Read the model definition and answer for the solid it produces. Units are mm, in the model's axes. A direction names the side the tool comes from. Coordinates: 2 decimals unless noted, no trailing zeros. Order: outer loops, then holes, each group sorted by start corner. A loop starts at its lowest first (then second) coordinate and runs counter-clockwise, first axis right, second up. Notation, with made-up numbers: (25.5, 63.5) -> (75.5, 63.5) arc R29 cw to (75.5, 86.5) -> close; hole circle Ø5 at (68.5, 51.25). An arc over 180 degrees is marked (long way). Return JSON: item names as keys, results as strings. Group by question number.
```python
from build123d import *

# Parameters (mm, degrees)
ESQUISSE1_R             = 65
DISQUE_DEPTH            = 3
ESQUISSE3_W             = 30.466369815
ESQUISSE3_H             = 200
COT_S_DEPTH             = 4
D_GAGEMENT_M42_D        = 4.5
ESQUISSE15_W            = 89.863216067
ESQUISSE15_H            = 32.096215679
ENL_V_MAT_EXTRU_1_DEPTH = 4
EMPLACEMENT_COMPOS_W    = 48
EMPLACEMENT_COMPOS_H    = 19
EMPLACEMENT_COMPOS_W_2  = 65
EMPLACEMENT_COMPOS_W_3  = 120.200529509
EMPLACEMENT_COMPOS_H_2  = 30.626013932
ENL_V_MAT_EXTRU_2_DEPTH = 4
CONG_1_R                = 8
D_GAGEMENT_M3_51_D      = 3.9
D_GAGEMENT_M3_51_DEPTH  = 3
D_GAGEMENT_M3_51_TIP    = 1.171678207
ESQUISSE19_W            = 20.5
ESQUISSE19_H            = 24.73475383
ENL_V_MAT_EXTRU_3_DEPTH = 4
ESQUISSE22_W            = 15
ESQUISSE22_H            = 22.73475383
ENL_V_MAT_EXTRU_4_DEPTH = 4


with BuildPart() as part:
    # Esquisse1 → disque (new body)
    with BuildSketch(Plane(origin=(0, 0, 0), x_dir=(1, 0, 0), z_dir=(0, 1, 0))):
        Circle(ESQUISSE1_R)
    extrude(amount=DISQUE_DEPTH)

    # Esquisse3 → cotés (cut, through all)
    with BuildSketch(Plane(origin=(0, 3, 0), x_dir=(1, 0, 0), z_dir=(0, 1, 0))):
        with Locations((-55.233184908, 0)):
            Rectangle(ESQUISSE3_W, ESQUISSE3_H)
        with Locations((55.233184908, 0)):
            Rectangle(ESQUISSE3_W, ESQUISSE3_H)
    extrude(amount=-COT_S_DEPTH, mode=Mode.SUBTRACT)

    # Dégagement M42 (through all)
    with Locations(Plane(origin=(0, 3, 0), x_dir=(1, 0, 0), z_dir=(0, 1, 0))):
        with Locations((-32.5, 42.5), (32.5, 42.5), (32.5, -42.5), (-32.5, -42.5)):
            Hole(D_GAGEMENT_M42_D / 2)

    # Esquisse15 → Enlèv. mat.-Extru.1 (cut, through all)
    with BuildSketch(Plane.XZ):
        with Locations((-4.931608034, 67.282861669)):
            Rectangle(ESQUISSE15_W, ESQUISSE15_H)
    extrude(amount=-ENL_V_MAT_EXTRU_1_DEPTH, mode=Mode.SUBTRACT)

    # emplacement compos → Enlèv. mat.-Extru.2 (cut, through all)
    with BuildSketch(Plane(origin=(0, 0, 0), x_dir=(-1, 0, 0), z_dir=(0, -1, 0))):
        with Locations((0, 38.367376915)):
            Rectangle(EMPLACEMENT_COMPOS_W, EMPLACEMENT_COMPOS_H)
        with Locations((0, 16)):
            Rectangle(EMPLACEMENT_COMPOS_W_2, EMPLACEMENT_COMPOS_H)
        with Locations((-20.100264755, 66.547760796)):
            Rectangle(EMPLACEMENT_COMPOS_W_3, EMPLACEMENT_COMPOS_H_2)
    extrude(amount=-ENL_V_MAT_EXTRU_2_DEPTH, mode=Mode.SUBTRACT)

    # Congé1
    cong_1_edges = [part.edges().sort_by_distance(p)[0] for p in [
        (40, 1.5, -51.23475383),
        (40, 1.5, 51.23475383),
        (-40, 1.5, 51.23475383),
        (-40, 1.5, -51.23475383),
    ]]
    fillet(cong_1_edges, radius=CONG_1_R)

    # Dégagement M3.51
    with Locations(Plane(origin=(0, 3, 0), x_dir=(1, 0, 0), z_dir=(0, 1, 0))):
        with Locations((-7.5, -28.23475383), (7.5, -28.23475383), (7.5, -43.23475383), (-7.5, -43.23475383)):
            Hole(D_GAGEMENT_M3_51_D / 2, depth=D_GAGEMENT_M3_51_DEPTH)
            with Locations((0, 0, -(D_GAGEMENT_M3_51_DEPTH + D_GAGEMENT_M3_51_TIP / 2))):  # 118° drill point
                Cone(0, D_GAGEMENT_M3_51_D / 2, D_GAGEMENT_M3_51_TIP, mode=Mode.SUBTRACT)

    # Esquisse19 → Enlèv. mat.-Extru.3 (cut, through all)
    with BuildSketch(Plane(origin=(0, 3, 0), x_dir=(1, 0, 0), z_dir=(0, 1, 0))):
        with Locations((-22.75, -10.867376915)):
            Rectangle(ESQUISSE19_W, ESQUISSE19_H)
    enl_v_mat_extru_3 = extrude(amount=-ENL_V_MAT_EXTRU_3_DEPTH, mode=Mode.SUBTRACT)

    # Symétrie1: Enlèv. mat.-Extru.3 across plane
    add(enl_v_mat_extru_3.mirror(Plane.ZY), mode=Mode.SUBTRACT)

    # Esquisse22 → Enlèv. mat.-Extru.4 (cut, through all)
    with BuildSketch(Plane(origin=(0, 3, 0), x_dir=(1, 0, 0), z_dir=(0, 1, 0))):
        with Locations((0, -9.867376915)):
            Rectangle(ESQUISSE22_W, ESQUISSE22_H)
    extrude(amount=-ENL_V_MAT_EXTRU_4_DEPTH, mode=Mode.SUBTRACT)


solid = part.part
```
1. Find section D-D on z = -10. Determine the outline of the cut face in (x, y).
2. Find section B-B on z = 6. Determine the outline of the cut face in (x, y).
3. Find section C-C on x = 20.5. Determine the outline of the cut face in (y, z), and give its area (3 significant figures).
4. Find section A-A on z = -32.5. Determine the outline of the cut face in (x, y).
5. Given pin 1 (2.5 mm diameter, centred on x = 32.5, z = 42.5, fed in from +Y), flat-ended and moving along its own axis, determine where the tip first touches the part or whether it passes through.
6. Which of the six approach directions +Z, -Z, +X, -X, +Y, -Y give full straight-line access (tool end or side, diameter ignored) to faces 1 (the face through (23, 2, -1.5)), 2 (the face through (37.594, 1.479, -48.953))?
7. For a pull along Z with two mould halves and no side action, classify faces 3 (the face through (-37.72, 1.48, 48.83)), 4 (the face through (-33.71, 1.479, 40.603)), 5 (the face through (-9, 3, 11)), 6 (the face through (7.5, 2, 10)) as released by +Z, released by -Z, zero draft, split by the parting line, or undercut.
8. Straight lines are drawn through the part: L1, parallel to X at y = 1.3, z = 9.5; L2, parallel to Z at x = -12, y = 0.85; L3, parallel to Z at x = -17, y = 2.75. For each, find the intervals that lie inside material, in ascending order.
Result:
{
 "1": {"outline": "(-40, 0) -> (-32.5, 0) -> (-32.5, 3) -> (-40, 3) -> close; (32.5, 0) -> (40, 0) -> (40, 3) -> (32.5, 3) -> close"},
 "2": {"outline": "(-40, 0) -> (-33, 0) -> (-33, 3) -> (-40, 3) -> close; (-12.5, 0) -> (-7.5, 0) -> (-7.5, 3) -> (-12.5, 3) -> close; (7.5, 0) -> (12.5, 0) -> (12.5, 3) -> (7.5, 3) -> close; (33, 0) -> (40, 0) -> (40, 3) -> (33, 3) -> close"},
 "3": {"outline": "(0, -51.23) -> (3, -51.23) -> (3, -47.87) -> (0, -47.87) -> close; (0, -28.87) -> (3, -28.87) -> (3, -25.5) -> (0, -25.5) -> close; (0, -6.5) -> (3, -6.5) -> (3, -1.5) -> (0, -1.5) -> close; (0, 23.23) -> (3, 23.23) -> (3, 51.23) -> (0, 51.23) -> close", "area": "119 mm^2"},
 "4": {"outline": "(-40, 0) -> (-24, 0) -> (-24, 3) -> (-40, 3) -> close; (24, 0) -> (40, 0) -> (40, 3) -> (24, 3) -> close"},
 "5": {"pin 1": "through"},
 "6": {"face 1": "+Y, -Y", "face 2": "-Z, +X, +Y, -Y"},
 "7": {"face 3": "released by +Z", "face 4": "undercut", "face 5": "zero draft", "face 6": "undercut"},
 "8": {"L1": "-40 to -33, -12.5 to -7.5, 7.5 to 12.5, 33 to 40", "L2": "-51.23 to -47.87, -28.87 to -25.5, -6.5 to 51.23", "L3": "-51.23 to -47.87, -28.87 to -25.5, -6.5 to -1.5, 23.23 to 51.23"}
}
